from build123d import *

# Parameters (mm, degrees)
BOSS_EXTRUDE1_DEPTH  = 381
CUT_EXTRUDE1_DEPTH   = 51.8
CUT_EXTRUDE3_DEPTH   = 26.4
M3_CLEARANCE_HOLE1_D = 3.4


with BuildPart() as part:
    # Sketch1 → Boss-Extrude1 (new body)
    with BuildSketch(Plane.XY):
        Polygon((-25.4, 0), (25.4, 0), (25.4, 25.4), (22.225, 25.4), (22.225, 3.175), (-22.225, 3.175), (-22.225, 25.4), (-25.4, 25.4), align=None)
    extrude(amount=BOSS_EXTRUDE1_DEPTH)

    # Sketch2 → Cut-Extrude1 (cut, through all)
    with BuildSketch(Plane(origin=(25.4, 0, 0), x_dir=(0, 0, -1), z_dir=(1, 0, 0))):
        Polygon((-381, 0), (-355.6, 25.4), (-381, 25.4), align=None)
        Polygon((0, 0), (0, 25.4), (-25.4, 25.4), align=None)
    extrude(amount=-CUT_EXTRUDE1_DEPTH, mode=Mode.SUBTRACT)

    # Sketch4 → Cut-Extrude3 (cut, through all)
    with BuildSketch(Plane.XZ):
        with BuildLine():
            Line((-13.97, 276.86), (13.97, 276.86))
            ThreePointArc((13.97, 276.86), (17.145, 273.685), (20.32, 276.86))
            Line((20.32, 276.86), (20.32, 304.8))
            ThreePointArc((20.32, 304.8), (17.145, 307.975), (13.97, 304.8))
            Line((13.97, 304.8), (-13.97, 304.8))
            ThreePointArc((-13.97, 304.8), (-17.145, 307.975), (-20.32, 304.8))
            Line((-20.32, 304.8), (-20.32, 276.86))
            ThreePointArc((-20.32, 276.86), (-17.145, 273.685), (-13.97, 276.86))
        make_face()
        with BuildLine():
            Line((-20.32, 104.14), (-20.32, 76.2))
            ThreePointArc((-20.32, 76.2), (-17.145, 73.025), (-13.97, 76.2))
            Line((-13.97, 76.2), (13.97, 76.2))
            ThreePointArc((13.97, 76.2), (17.145, 73.025), (20.32, 76.2))
            Line((20.32, 76.2), (20.32, 104.14))
            ThreePointArc((20.32, 104.14), (17.145, 107.315), (13.97, 104.14))
            Line((13.97, 104.14), (-13.97, 104.14))
            ThreePointArc((-13.97, 104.14), (-17.145, 107.315), (-20.32, 104.14))
        make_face()
    extrude(amount=-CUT_EXTRUDE3_DEPTH, mode=Mode.SUBTRACT)

    # M3 Clearance Hole1 (through all)
    with Locations(Plane(origin=(-25.4, 12.7, 50.8), x_dir=(0, -1, 0), z_dir=(-1, 0, 0))):
        with Locations((0, 0), (0, 139.7), (0, 279.4)):
            Hole(M3_CLEARANCE_HOLE1_D / 2)


solid = part.part
CAD build for the part. Positions are in the model's coordinates, mm. A direction names the side the tool comes from. Round coordinates to 2 decimals unless told otherwise and drop trailing zeros. Loops run counter-clockwise (first coordinate to the right, second up) from the corner with the lowest first, then second, coordinate; pieces in that order, holes last.
(1) Drop flat-ended pins along their axis: pin 1 (3 mm diameter, centred on y = 12.7, z = 50.8, fed in from +X); pin 2 (2.5 mm diameter, centred on x = -1, y = 2.5, fed in from -Z); pin 3 (10 mm diameter, centred on x = 15.5, z = 114, fed in from -Y); pin 4 (6 mm diameter, centred on x = 17.5, z = 126.5, fed in from +Y) (3 decimals). Give the stop position or say it passes through.
(2) Wall check: line 1 along Y through (x, z) = (23, 190.5); line 2 along X through (y, z) = (5, 351) (3 decimals); line 3 along Z through (x, y) = (24.4, 12.7). Give the ranges that are in metal, low to high.
(3) Cut at C-C (z = 263). Give the cut face in (x, y) (3 decimals).
(4) Cut at A-A (y = 17.75). Give the cut face in (x, z) (3 decimals), plus the area to 3 significant figures.
(5) Cut at B-B (x = 7). Give the cut face in (y, z) (3 decimals), plus the area to 3 significant figures.
(6) Which spindle directions (+Z, -Z, +X, -X, +Y, -Y) get a long thin tool onto all of the face, cutting with end or side? Do faces 5 (the flat face through (0, 0, 188)), 6 (the flat face through (-22.225, 14, 188)). Say none if no direction does.
(7) Two-plate mould, pull along X, no slides. Class faces 1 (the flat face through (0, 3.175, 188)), 2 (the flat face through (25.4, 13, 188)), 3 (the flat face through (0, 2, 379)), 4 (the flat face through (22.225, 14, 188)): +X half, -X half, draft (parallel to the pull), parting line (faces both ways), or undercut.
Findings below:
1. pin 1: passes through
1. pin 2: stops at z = 1.25
1. pin 3: stops at y = 0
1. pin 4: stops at y = 3.175
2. line 1: y = 0 to 11, 14.4 to 25.4
2. line 2: x = -25.4 to -22.225, 22.225 to 25.4
2. line 3: z = 12.7 to 49.1, 52.5 to 188.8, 192.2 to 328.5, 331.9 to 368.3
3. outline: (-25.4, 0) - (25.4, 0) - (25.4, 25.4) - (22.225, 25.4) - (22.225, 3.175) - (-22.225, 3.175) - (-22.225, 25.4) - (-25.4, 25.4) - close
4. outline: (-25.4, 17.75) - (-22.225, 17.75) - (-22.225, 363.25) - (-25.4, 363.25) - close; (22.225, 17.75) - (25.4, 17.75) - (25.4, 363.25) - (22.225, 363.25) - close
4. area: 2,190 mm2
5. outline: (0, 0) - (3.175, 3.175) - (3.175, 76.2) - (0, 76.2) - close; (0, 104.14) - (3.175, 104.14) - (3.175, 276.86) - (0, 276.86) - close; (0, 304.8) - (3.175, 304.8) - (3.175, 377.825) - (0, 381) - close
5. area: 1,020 mm2
6. face 5: +Z, -Z, +X, -X, -Y
6. face 6: +Z, -Z, +Y
7. face 1: undercut
7. face 2: +X half
7. face 3: draft
7. face 4: undercut
